Geometry check sheet. Reference: the model listing, model coordinates, mm. A direction names the side the tool comes from. Give positions to 0.01 mm unless a question says otherwise; leave off trailing zeros. Write each loop counter-clockwise with the first axis right and the second up, starting at its lowest first coordinate (ties: lowest second). Pieces come first, ordered by that corner, then holes. Notation, with made-up numbers: (64, -26) -> (120, -26) arc R21 cw to (120, -17) -> close; hole circle Ø5 at (-30.75, 17). An arc over 180 degrees is marked (long way). Write item = value, one per line. Start each with the question number.
1. Cross-section at D-D, the plane x = -8.5. Record the cut outline in (y, z), plus the area to 3 significant figures.
2. Cross-section at B-B, the plane z = 15. Record the cut outline in (x, y), plus the area to 3 significant figures.
3. Thickness scan on line 1 along Z through (x, y) = (-7.5, 16.5); line 2 along X through (y, z) = (19, 14); line 3 along Z through (x, y) = (-15, -6.5). Record the ranges inside material, lowest first.
4. Cross-section at A-A, the plane z = 24. Record the cut outline in (x, y), plus the area to 3 significant figures.
5. Depth check by flat-ended pin: P1, Ø1.7, axis at x = 22, y = -11.5, coming from the +Z side; P2, Ø5, axis at y = 20.5, z = 7.5, coming from the -X side; P3, Ø12, axis at x = -9.5, z = 20.5, coming from the -Y side; P4, Ø1.5, axis at x = -12.5, z = 4.5, coming from the +Y side. Enter the tip coordinate at first touch or a pass-through.
6. Mould release check, pull along X, two halves, no side actions. Record for faces 1 (the cylindrical face through (-19.53, -14.09, 1.91)), 2 (the cylindrical face through (19.53, -14.09, 1.91)), 3 (the flat face through (20.483, -9.517, 14.79)), 4 (the cylindrical face through (0.07, 16.17, 2.56)): pulls with the +X half, pulls with the -X half, needs draft (parallel to the pull), parting line crosses it, or undercut.
7. Cross-section at C-C, the plane y = 16.5. Record the cut outline in (x, z).
8. Set-up check for faces 5 (the flat face through (0, 17.427, 17)), 6 (the flat face through (0, 0, 2)), 7 (the flat face through (15.1, -8.7, 17.3)): record each of +Z, -Z, +X, -X, +Y, -Y from which the full face is reachable in a straight line by a thin tool's end or side.
```python
from build123d import *

# Parameters (mm, degrees)
F5_DEPTH = 30
F6_DEPTH = 20
F0_COUNT = 3
F1_DEPTH = 2
F2_R     = 3


# Not quite as in the source:
# - a feature names something its author has since deleted; it is built from what else it names


with BuildPart() as f5:
    # F4 (on Top) → F5 (new body)
    with BuildSketch(Plane.XY):
        with BuildLine():
            ThreePointArc((2, 22.9128784748), (0, 23), (-2, 22.9128784748))
            Line((-2, 22.9128784748), (-2, 17.4271763038))
            Line((-2, 17.4271763038), (2, 17.4271763038))
            Line((2, 17.4271763038), (2, 22.9128784748))
        make_face()
    extrude(amount=F5_DEPTH)

    # F4 (on Top) → F6 (join)
    with BuildSketch(Plane.XY):
        with BuildLine():
            Line((2, 24.4271763038), (2, 27.4271763038))
            Line((2, 27.4271763038), (-2, 27.4271763038))
            Line((-2, 27.4271763038), (-2, 22.9128784748))
            ThreePointArc((-2, 22.9128784748), (0, 23), (2, 22.9128784748))
            Line((2, 22.9128784748), (2, 24.4271763038))
        make_face()
        with BuildLine():
            Line((-2, 27.4271763038), (2, 27.4271763038))
            ThreePointArc((2, 27.4271763038), (0, 27.5), (-2, 27.4271763038))
        make_face()
    extrude(amount=F6_DEPTH)


with BuildPart() as f0_1:
    # F0: instance of F5
    add(f5.part.rotate(Axis((0, 0, 0), (0, 0, 1)), 1 * 360 / F0_COUNT))


with BuildPart() as f0_2:
    # F0: instance of F5
    add(f5.part.rotate(Axis((0, 0, 0), (0, 0, 1)), 2 * 360 / F0_COUNT))


with BuildPart() as f5_1:
    add(f5.part)

    add(f0_1.part)  # F1 merges F0_1

    add(f0_2.part)  # F1 merges F0_2
    # F4 (on Top) → F1 (join)
    with BuildSketch(Plane.XY):
        with BuildLine():
            ThreePointArc((2, 22.9128784748), (0, 23), (-2, 22.9128784748))
            Line((-2, 22.9128784748), (-2, 17.4271763038))
            Line((-2, 17.4271763038), (2, 17.4271763038))
            Line((2, 17.4271763038), (2, 22.9128784748))
        make_face()
        with BuildLine():
            Line((-2, 17.4271763038), (-2, 22.9128784748))
            ThreePointArc((-2, 22.9128784748), (-15.5402702679, -16.9558249578), (23, 0))
            ThreePointArc((23, 0), (16.9558249578, 15.5402702679), (2, 22.9128784748))
            Line((2, 22.9128784748), (2, 17.4271763038))
            Line((2, 17.4271763038), (-2, 17.4271763038))
        make_face()
    extrude(amount=F1_DEPTH)

    # F2
    f2_edges = [f5_1.edges().sort_by_distance(p)[0] for p in [
        (-2, 20.170027, 2),
        (0, 17.427176, 2),
        (2, 20.170027, 2),
        (16.467756, -11.817065, 2),
        (15.092377, -8.713588, 2),
        (18.467756, -8.352963, 2),
        (-18.467756, -8.352963, 2),
        (-15.092377, -8.713588, 2),
        (-16.467756, -11.817065, 2),
        (-2, 22.912878, 1),
        (-20.843135, -9.724388, 1),
        (2, 22.912878, 1),
        (20.843135, -9.724388, 1),
        (18.843135, -13.18849, 1),
        (-18.843135, -13.18849, 1),
    ]]
    fillet(f2_edges, radius=F2_R)


solid = f5_1.part
```
Answers:
q1.outline = (-21.37, 0) -> (21.37, 0) -> (21.37, 2) -> (-21.37, 2) -> close
q1.area = 85.5 mm^2
q2.outline = (-24.75, -11.98) arc R27.5 ccw to (-22.75, -15.45) -> (-14.09, -10.45) -> (-16.09, -6.98) -> close; (-2, 17.43) -> (2, 17.43) -> (2, 27.43) arc R27.5 ccw to (-2, 27.43) -> close; (14.09, -10.45) -> (22.75, -15.45) arc R27.5 ccw to (24.75, -11.98) -> (16.09, -6.98) -> close
q2.area = 121 mm^2
q3.line_1 = 0 to 2
q3.line_2 = -2 to 2
q3.line_3 = 0 to 2.61
q4.outline = (-20.84, -9.72) arc R23 ccw to (-18.84, -13.19) -> (-14.09, -10.45) -> (-16.09, -6.98) -> close; (-2, 17.43) -> (2, 17.43) -> (2, 22.91) arc R23 ccw to (-2, 22.91) -> close; (14.09, -10.45) -> (18.84, -13.19) arc R23 ccw to (20.84, -9.72) -> (16.09, -6.98) -> close
q4.area = 66.5 mm^2
q5.P1 = 20
q5.P2 = -2
q5.P3 = -11.26
q5.P4 = through
q6.face_1 = undercut
q6.face_2 = undercut
q6.face_3 = pulls with the +X half
q6.face_4 = needs draft
q7.outline = (-16.02, 0) -> (16.02, 0) -> (16.02, 2) -> (5, 2) arc R3 cw to (2.93, 2.83) -> (-2.93, 2.83) arc R3 cw to (-5, 2) -> (-16.02, 2) -> close
q8.face_5 = +Z, +X, -X, -Y
q8.face_6 = +Z
q8.face_7 = +Z, +Y
